```python
from build123d import *

# Parameters (mm, degrees)
F0_R     = 58
F1_DEPTH = 30
F2_T     = -3
F3_R     = 2
F5_D     = 8
F7_D     = 5


with BuildPart() as f1:
    # F0 (on Front) → F1 (new body)
    with BuildSketch(Plane.XZ):
        Circle(F0_R)
    extrude(amount=F1_DEPTH)

    # F2
    f2_openings = [f1.faces().sort_by_distance(p)[0] for p in [
        (0, 0, 0),
    ]]
    offset(amount=F2_T, openings=f2_openings)

    # F3
    f3_edges = [f1.edges().sort_by_distance(p)[0] for p in [
        (-58, -30, 0),
    ]]
    fillet(f3_edges, radius=F3_R)

    # F5 (through all)
    with Locations(Plane.XZ.offset(30)):
        with Locations((0, 0)):
            Hole(F5_D / 2)

    # F7 (through all)
    with Locations(Plane.XZ.offset(30)):
        with Locations((0, 25), (0, 50), (-23.776413, 7.725425), (-47.552826, 15.45085), (-29.389263, -40.45085), (-14.694631, -20.225425), (14.694631, -20.225425), (29.389263, -40.45085), (23.776413, 7.725425), (47.552826, 15.45085)):
            Hole(F7_D / 2)


solid = f1.part
```
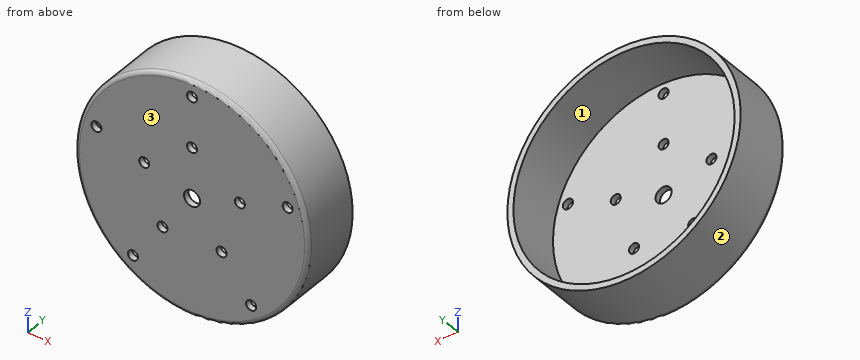
Model file for the job. Use its own axes, mm. Face numbers are marked on the shaded views. Coordinates: 2 decimals unless noted, no trailing zeros. Write each loop counter-clockwise with the first axis right and the second up, starting at its lowest first coordinate (ties: lowest second). Pieces come first, ordered by that corner, then holes. Notation, with made-up numbers: (-28.5, -16) - (30.5, -16) arc R11 ccw to (30.5, 4) - close; hole circle Ø11 at (33, 58). An arc over 180 degrees is marked (long way). Use a Markdown table: item, result. Add a question column.
Item 1: Drop flat-ended pins along their axis: pin 1 (1.5 mm diameter, centred on y = -21, z = -6.5, fed in from +X); pin 2 (1.5 mm diameter, centred on x = 12, y = -12.5, fed in from -Z); pin 3 (1.5 mm diameter, centred on y = -11.5, z = -36.5, fed in from -X); pin 4 (8 mm diameter, centred on x = 0, z = 50, fed in from -Y). Give the stop position or say it passes through.
Item 2: Drill centre lines: line 1 along Z through (x, y) = (-1, -23.25); line 2 along Y through (x, z) = (-15, 29); line 3 along Z through (x, y) = (-7, -9). Where is each one in solid material? Low to high.
Item 3: Band-saw the part on C-C, the plane y = -14.5. Write the cut outline in (x, z), and give its area (4 significant figures).
Item 4: Two-plate mould, pull along Z, no slides. Class the marked faces 1, 2 and 3: pulls with the +Z half, pulls with the -Z half, needs draft (parallel to the pull), parting line crosses it, or undercut.
Item 5: Band-saw the part on A-A, the plane z = 0. Write the cut outline in (x, y).
Item 6: Band-saw the part on B-B, the plane x = 0. Write the cut outline in (y, z), and give its area (3 significant figures).
A:
| question | item | result |
|---|---|---|
| 1 | pin 1 | stops at x = 57.71 |
| 1 | pin 2 | stops at z = -56.9 |
| 1 | pin 3 | stops at x = -45.67 |
| 1 | pin 4 | stops at y = -30 |
| 2 | line 1 | z = -57.99 to -54.99, 54.99 to 57.99 |
| 2 | line 2 | y = -30 to -27 |
| 2 | line 3 | z = -57.58 to -54.55, 54.55 to 57.58 |
| 3 | outline | circle Ø116 at (0, 0); hole circle Ø110 at (0, 0) |
| 3 | area | 1,065 mm² |
| 4 | face 1 | undercut |
| 4 | face 2 | parting line crosses it |
| 4 | face 3 | needs draft |
| 5 | outline | (-58, -28) arc R2 ccw to (-56, -30) - (-4, -30) - (-4, -27) - (-55, -27) - (-55, 0) - (-58, 0) - close; (4, -30) - (56, -30) arc R2 ccw to (58, -28) - (58, 0) - (55, 0) - (55, -27) - (4, -27) - close |
| 6 | outline | (-30, -56) arc R2 ccw to (-28, -58) - (0, -58) - (0, -55) - (-27, -55) - (-27, -4) - (-30, -4) - close; (-30, 4) - (-27, 4) - (-27, 22.5) - (-30, 22.5) - close; (-30, 27.5) - (-27, 27.5) - (-27, 47.5) - (-30, 47.5) - close; (-30, 52.5) - (-27, 52.5) - (-27, 55) - (0, 55) - (0, 58) - (-28, 58) arc R2 ccw to (-30, 56) - close |
| 6 | area | 454 mm² |
